Work out the finished part from the listing and answer in its coordinate system (mm). Face numbers are marked on the shaded views. Coordinates: 2 decimals unless noted, no trailing zeros. Loops run counter-clockwise (first coordinate to the right, second up) from the corner with the lowest first, then second, coordinate; pieces in that order, holes last. Notation, with made-up numbers: (-18.5, 37.25) -> (19.5, 37.25) arc R14 cw to (19.5, 47.25) -> close; hole circle Ø11 at (-14, 81.5). An arc over 180 degrees is marked (long way). Answer as CSV lines item,"result".
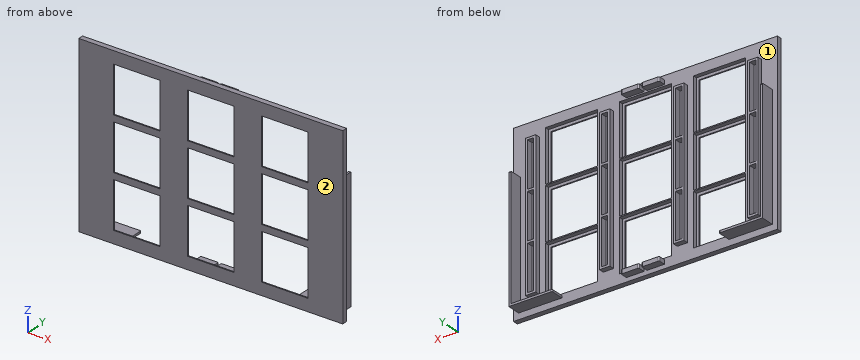
```python
from build123d import *

# Parameters (mm, degrees)
SKETCH2_W           = 128
SKETCH2_H           = 86
BOSS_EXTRUDE1_DEPTH = 2.5
SKETCH3_W           = 25.2
SKETCH3_H           = 25.2
SKETCH3_H_2         = 12.6
CUT_EXTRUDE1_DEPTH  = 2
SKETCH4_W           = 22.6
SKETCH4_H           = 22.6
CUT_EXTRUDE2_DEPTH  = 2.5
SKETCH5_W           = 5
SKETCH5_H           = 70
BOSS_EXTRUDE2_DEPTH = 2.5
SKETCH7_W           = 3
SKETCH7_H           = 22
CUT_EXTRUDE6_DEPTH  = 3
SKETCH9_W           = 8.5
SKETCH9_H           = 2
BOSS_EXTRUDE3_DEPTH = 6.5
CUT_EXTRUDE9_START  = 3.5
SKETCH10_W          = 8.5
SKETCH10_H          = 2
CUT_EXTRUDE9_DEPTH  = 74.877322259
FILLET1_R           = 0.5


with BuildPart() as part:
    # Sketch2 → Boss-Extrude1 (new body)
    with BuildSketch(Plane(origin=(0, 0, 0), x_dir=(1, 0, 0), z_dir=(0, 1, 0))):
        Rectangle(SKETCH2_W, SKETCH2_H)
    extrude(amount=-BOSS_EXTRUDE1_DEPTH)

    # Sketch3 → Cut-Extrude1 (cut)
    with BuildSketch(Plane(origin=(0, 0, 0), x_dir=(1, 0, 0), z_dir=(0, 1, 0))):
        with Locations((0, 25.7)):
            Rectangle(SKETCH3_W, SKETCH3_H)
        with Locations((35.9, 25.7)):
            Rectangle(SKETCH3_W, SKETCH3_H)
        with Locations((35.9, 6.3)):
            Rectangle(SKETCH3_W, SKETCH3_H_2)
        with Locations((35.9, -6.3)):
            Rectangle(SKETCH3_W, SKETCH3_H_2)
        with Locations((35.9, -25.7)):
            Rectangle(SKETCH3_W, SKETCH3_H)
        with Locations((0, 6.3)):
            Rectangle(SKETCH3_W, SKETCH3_H_2)
        with Locations((0, -6.3)):
            Rectangle(SKETCH3_W, SKETCH3_H_2)
        with Locations((0, -25.7)):
            Rectangle(SKETCH3_W, SKETCH3_H)
        with Locations((-35.9, 25.7)):
            Rectangle(SKETCH3_W, SKETCH3_H)
        with Locations((-35.9, 6.3)):
            Rectangle(SKETCH3_W, SKETCH3_H_2)
        with Locations((-35.9, -6.3)):
            Rectangle(SKETCH3_W, SKETCH3_H_2)
        with Locations((-35.9, -25.7)):
            Rectangle(SKETCH3_W, SKETCH3_H)
    extrude(amount=-CUT_EXTRUDE1_DEPTH, mode=Mode.SUBTRACT)

    # Sketch4 → Cut-Extrude2 (cut)
    with BuildSketch(Plane(origin=(0, 0, 0), x_dir=(1, 0, 0), z_dir=(0, 1, 0))):
        Rectangle(SKETCH4_W, SKETCH4_H)
        with Locations((0, 25.7)):
            Rectangle(SKETCH4_W, SKETCH4_H)
        with Locations((0, -25.7)):
            Rectangle(SKETCH4_W, SKETCH4_H)
        with Locations((35.9, -25.7)):
            Rectangle(SKETCH4_W, SKETCH4_H)
        with Locations((35.9, 0)):
            Rectangle(SKETCH4_W, SKETCH4_H)
        with Locations((35.9, 25.7)):
            Rectangle(SKETCH4_W, SKETCH4_H)
        with Locations((-35.9, -25.7)):
            Rectangle(SKETCH4_W, SKETCH4_H)
        with Locations((-35.9, 0)):
            Rectangle(SKETCH4_W, SKETCH4_H)
        with Locations((-35.9, 25.7)):
            Rectangle(SKETCH4_W, SKETCH4_H)
    extrude(amount=-CUT_EXTRUDE2_DEPTH, mode=Mode.SUBTRACT)

    # Sketch5 → Boss-Extrude2 (add)
    with BuildSketch(Plane(origin=(0, 0, 0), x_dir=(1, 0, 0), z_dir=(0, 1, 0))):
        with Locations((-53.85, 0)):
            Rectangle(SKETCH5_W, SKETCH5_H)
        with Locations((-17.95, 0)):
            Rectangle(SKETCH5_W, SKETCH5_H)
        with Locations((17.95, 0)):
            Rectangle(SKETCH5_W, SKETCH5_H)
        with Locations((53.85, 0)):
            Rectangle(SKETCH5_W, SKETCH5_H)
    extrude(amount=BOSS_EXTRUDE2_DEPTH)

    # Sketch7 → Cut-Extrude6 (cut)
    with BuildSketch(Plane(origin=(0, 2.5, 0), x_dir=(1, 0, 0), z_dir=(0, 1, 0))):
        with Locations((-17.95, 23)):
            Rectangle(SKETCH7_W, SKETCH7_H)
        with Locations((-17.95, 0)):
            Rectangle(SKETCH7_W, SKETCH7_H)
        with Locations((-17.95, -23)):
            Rectangle(SKETCH7_W, SKETCH7_H)
        with Locations((17.95, 23)):
            Rectangle(SKETCH7_W, SKETCH7_H)
        with Locations((17.95, 0)):
            Rectangle(SKETCH7_W, SKETCH7_H)
        with Locations((17.95, -23)):
            Rectangle(SKETCH7_W, SKETCH7_H)
        with Locations((53.85, 23)):
            Rectangle(SKETCH7_W, SKETCH7_H)
        with Locations((53.85, 0)):
            Rectangle(SKETCH7_W, SKETCH7_H)
        with Locations((-53.85, 23)):
            Rectangle(SKETCH7_W, SKETCH7_H)
        with Locations((-53.85, 0)):
            Rectangle(SKETCH7_W, SKETCH7_H)
        with Locations((-53.85, -23)):
            Rectangle(SKETCH7_W, SKETCH7_H)
        with Locations((53.85, -23)):
            Rectangle(SKETCH7_W, SKETCH7_H)
    extrude(amount=-CUT_EXTRUDE6_DEPTH, mode=Mode.SUBTRACT)

    # Sketch9 → Boss-Extrude3 (add)
    with BuildSketch(Plane(origin=(0, 0, 0), x_dir=(1, 0, 0), z_dir=(0, 1, 0))):
        Polygon((-61.5, -20), (-60.5, -20), (-60.5, 39), (-40.5, 39), (-40.5, 40), (-61.5, 40), align=None)
        Polygon((40.5, 40), (61.5, 40), (61.5, -20), (60.5, -20), (60.5, 39), (40.5, 39), align=None)
        with Locations((-5, 40)):
            Rectangle(SKETCH9_W, SKETCH9_H)
        with Locations((5, 40)):
            Rectangle(SKETCH9_W, SKETCH9_H)
        with Locations((-5, -40)):
            Rectangle(SKETCH9_W, SKETCH9_H)
        with Locations((5, -40)):
            Rectangle(SKETCH9_W, SKETCH9_H)
    extrude(amount=BOSS_EXTRUDE3_DEPTH)

    # Sketch10 → Cut-Extrude9 (cut, through all)
    with BuildSketch(Plane(origin=(0, 0, 0), x_dir=(1, 0, 0), z_dir=(0, 1, 0)).offset(CUT_EXTRUDE9_START)):
        with Locations((-5, 40)):
            Rectangle(SKETCH10_W, SKETCH10_H)
        with Locations((5, 40)):
            Rectangle(SKETCH10_W, SKETCH10_H)
        with Locations((-5, -40)):
            Rectangle(SKETCH10_W, SKETCH10_H)
        with Locations((5, -40)):
            Rectangle(SKETCH10_W, SKETCH10_H)
    extrude(amount=CUT_EXTRUDE9_DEPTH, mode=Mode.SUBTRACT)

    # Fillet1
    fillet1_edges = [part.edges().sort_by_distance(p)[0] for p in [
        (40.5, 6.5, -39.5),
        (61, 6.5, 20),
        (-61, 6.5, 20),
        (-40.5, 6.5, -39.5),
        (0.75, 3.5, -40),
        (9.25, 3.5, -40),
        (-9.25, 3.5, 40),
        (-0.75, 3.5, 40),
        (0.75, 3.5, 40),
        (9.25, 3.5, 40),
        (-9.25, 3.5, -40),
        (-0.75, 3.5, -40),
    ]]
    fillet(fillet1_edges, radius=FILLET1_R)


solid = part.part
```
(1) For a pull along X with two mould halves and no side action, classify the marked faces 1 and 2 as pulls with the +X half, pulls with the -X half, needs draft (parallel to the pull), parting line crosses it, or undercut.
Computed values:
face 1,"undercut"
face 2,"needs draft"
(2) Consider line 1 along Z through (x, y) = (28.5, -1); line 2 along X through (y, z) = (-1, 38); line 3 along X through (y, z) = (4.25, 2.5). Determine where each line is inside the solid, lowest interval first.
Computed values:
line 1,"-43 to -38.3, -13.1 to -12.6, 12.6 to 13.1, 38.3 to 43"
line 2,"-64 to -48.5, -23.3 to -12.6, 12.6 to 23.3, 48.5 to 64"
line 3,"-61.5 to -60.5, 60.5 to 61.5"
(3) A cutting plane is placed at B-B, the plane y = 1.25. Count the separate pieces of the cut face and the enclosed holes in it, and give its area (3 significant figures).
Computed values:
separate pieces,"10"
enclosed holes,"12"
area,"836 mm2"
(4) Flat-ended cylindrical pins translate along their axes: pin 1 Ø1.5 at (x, y) = (-18, 1.5) entering from -Z; pin 2 Ø4 at (y, z) = (5, -15) entering from +X; pin 3 Ø0.9 at (y, z) = (1.5, 24.5) entering from -X; pin 4 Ø2 at (y, z) = (5, 31.5) entering from -X. Find the tip coordinate at first contact, or state that the pin passes through.
Computed values:
pin 1,"z = -35"
pin 2,"x = 61.5"
pin 3,"x = -56.35"
pin 4,"through"
(5) A cutting plane is placed at A-A, the plane x = -28.5. Write down the section's boundary in (y, z).
Computed values:
outline,"(-2.5, -43) -> (0, -43) -> (0, -38.3) -> (-2, -38.3) -> (-2, -37) -> (-2.5, -37) -> close; (-2.5, -14.4) -> (-2, -14.4) -> (-2, -13.1) -> (0, -13.1) -> (0, -12.6) -> (-2, -12.6) -> (-2, -11.3) -> (-2.5, -11.3) -> close; (-2.5, 11.3) -> (-2, 11.3) -> (-2, 12.6) -> (0, 12.6) -> (0, 13.1) -> (-2, 13.1) -> (-2, 14.4) -> (-2.5, 14.4) -> close; (-2.5, 37) -> (-2, 37) -> (-2, 38.3) -> (0, 38.3) -> (0, 43) -> (-2.5, 43) -> close"
